Verification items for the finished model (mm, model axes). A direction names the side the tool comes from. Give positions to 0.01 mm unless a question says otherwise; leave off trailing zeros. Order: outer loops, then holes, each group sorted by start corner. A loop starts at its lowest first (then second) coordinate and runs counter-clockwise, first axis right, second up. Notation, with made-up numbers: (30, 3) -> (67, 3) arc R29 ccw to (67, 31) -> close; hole circle Ø9 at (-2, -28.75). An arc over 180 degrees is marked (long way). One line per question, with ' | ' between items. Start each with the question number.
Q1. Section check A-A on z = 18.75. Record the cut outline in (x, y), plus the area to 3 significant figures.
Q2. Mould release check, pull along Y, two halves, no side actions. Record for faces 3 (the flat face through (15, -12.7, 13)), 4 (the flat face through (19, 0, 0)), 5 (the flat face through (13, 0, 12.7)), 6 (the flat face through (13, 6.35, 19)): released by +Y, released by -Y, zero draft, split by the parting line, or undercut.
Q3. Go/stop test with flat-tipped pins: pin 1 (1.5 mm diameter, centred on x = 9, y = -4, fed in from +Z); pin 2 (2 mm diameter, centred on y = 3, z = 14.5, fed in from -X). Record where each tip stops, or that it passes through.
Q4. Section check C-C on z = 9. Record the cut outline in (x, y), plus the area to 3 significant figures.
Q5. Section check B-B on x = 13.5. Record the cut outline in (y, z).
Q6. Access from +Z, -Z, +X, -X, +Y, -Y to the whole of each face (thin tool, end or side, straight path). Record for faces 1 (the flat face through (30.558, -0.178, 10.056)), 2 (the flat face through (13, -6.35, 19)).
Q7. Section check D-D on y = 7. Record the cut outline in (x, z).
Q8. Material ranges on probe 1 along Y at (x, z) = (11.5, 21.5); probe 2 along Z at (x, y) = (3, -3.5), recorded low to high. Write a range as [from, to].
from build123d import *

# Parameters (mm, degrees)
F0_W     = 38.1
F0_H     = 25.4
F1_DEPTH = 12.7
F3_DEPTH = 25.4
F4_W     = 12.7
F4_H     = 12.7
F5_DEPTH = 25.4


with BuildPart() as f1:
    # F0 (on Front) → F1 (new body, symmetric)
    with BuildSketch(Plane.XZ):
        with Locations((19.05, 12.7)):
            Rectangle(F0_W, F0_H)
    extrude(amount=F1_DEPTH, both=True)

    # F2 (on face) → F3 (cut)
    with BuildSketch(Plane.XZ.offset(12.7)):
        Polygon((38.1, 25.4), (19.05, 25.4), (38.1, 0), align=None)
    extrude(amount=-F3_DEPTH, mode=Mode.SUBTRACT)

    # F4 (on Right) → F5 (cut)
    with BuildSketch(Plane.YZ):
        with Locations((0, 19.05)):
            Rectangle(F4_W, F4_H)
    extrude(amount=F5_DEPTH, mode=Mode.SUBTRACT)


solid = f1.part
Filled in:
1) outline: (0, -12.7) -> (24.04, -12.7) -> (24.04, -6.35) -> (0, -6.35) -> close; (0, 6.35) -> (24.04, 6.35) -> (24.04, 12.7) -> (0, 12.7) -> close | area: 305 mm²
2) face 3: released by -Y | face 4: zero draft | face 5: undercut | face 6: undercut
3) pin 1: z = 12.7 | pin 2: x = 25.4
4) outline: (0, -12.7) -> (31.35, -12.7) -> (31.35, 12.7) -> (0, 12.7) -> close | area: 796 mm²
5) outline: (-12.7, 0) -> (12.7, 0) -> (12.7, 25.4) -> (6.35, 25.4) -> (6.35, 12.7) -> (-6.35, 12.7) -> (-6.35, 25.4) -> (-12.7, 25.4) -> close
6) face 1: +Z, +X, +Y, -Y | face 2: +Z, -X
7) outline: (0, 0) -> (38.1, 0) -> (19.05, 25.4) -> (0, 25.4) -> close
8) probe 1: [-12.7, -6.35], [6.35, 12.7] | probe 2: [0, 12.7]
